Here's how the part is built. I have some questions about the finished solid (model axes, mm). A direction names the side the tool comes from. Round coordinates to 2 decimals unless told otherwise and drop trailing zeros. Order: outer loops, then holes, each group sorted by start corner. A loop starts at its lowest first (then second) coordinate and runs counter-clockwise, first axis right, second up. Notation, with made-up numbers: (53.25, 74.25) -> (111.25, 74.25) arc R10 ccw to (111.25, 91.25) -> close; hole circle Ø3 at (34.25, 29). An arc over 180 degrees is marked (long way). Answer in a Markdown table with one row per item.
```python
from build123d import *

# Parameters (mm, degrees)
F0_W     = 82
F0_H     = 25
F1_DEPTH = 4.5
F2_T     = -1.75
F3_W     = 70.6
F3_H     = 19.5
F4_DEPTH = 50.8
F5_W     = 1
F5_H     = 1.75
F6_DEPTH = 19.49958
F7_W     = 15.24
F7_H     = 5.5
F8_DEPTH = 1.75006


with BuildPart() as f1:
    # F0 (on Front) → F1 (new body)
    with BuildSketch(Plane.XZ):
        Rectangle(F0_W, F0_H)
    extrude(amount=F1_DEPTH)

    # F2
    f2_openings = [f1.faces().sort_by_distance(p)[0] for p in [
        (0, -2.25, 12.5),
    ]]
    offset(amount=F2_T, openings=f2_openings)

    # F3 (on face) → F4 (cut)
    with BuildSketch(Plane.XZ.offset(4.5)):
        with Locations((0, 2.75)):
            Rectangle(F3_W, F3_H)
    extrude(amount=-F4_DEPTH, mode=Mode.SUBTRACT)

    # F5 (on face) → F6 (cut)
    with BuildSketch(Plane.XY.offset(12.5)):
        with Locations((-35.8, -0.875)):
            Rectangle(F5_W, F5_H)
    extrude(amount=-F6_DEPTH, mode=Mode.SUBTRACT)

    # F7 (on face) → F8 (cut)
    with BuildSketch(Plane.XZ.offset(4.5)):
        with Locations((26.41, -9.75)):
            Rectangle(F7_W, F7_H)
    extrude(amount=-F8_DEPTH, mode=Mode.SUBTRACT)


solid = f1.part
```
1. For faces 4 (the face through (34.03, -4, -10)), 5 (the face through (-19, -2.75, -8)), 6 (the face through (-9, -4, -7)), 7 (the face through (-36.3, -1, 3)), which set-ups out of +Z, -Z, +X, -X, +Y, -Y let a thin tool reach every point of the face, with its end or its side?
Numbers:
| item | result |
|---|---|
| face 4 | +Z, -Z, -Y |
| face 5 | +Z |
| face 6 | +Z, +Y, -Y |
| face 7 | +Z, +Y |
2. Suppose I cut it at A-A on z = -2.25. Write out the boundary of the cut face in (x, y).
Numbers:
| item | result |
|---|---|
| outline | (-41, -4.5) -> (-35.3, -4.5) -> (-35.3, -2.75) -> (-39.25, -2.75) -> (-39.25, -1.75) -> (-36.3, -1.75) -> (-36.3, 0) -> (-41, 0) -> close; (35.3, -4.5) -> (41, -4.5) -> (41, 0) -> (35.3, 0) -> (35.3, -1.75) -> (39.25, -1.75) -> (39.25, -2.75) -> (35.3, -2.75) -> close |
3. Suppose I cut it at B-B on x = 1.5. Write out the boundary of the cut face in (y, z), then the cut area to 3 significant figures.
Numbers:
| item | result |
|---|---|
| outline | (-4.5, -12.5) -> (0, -12.5) -> (0, -7) -> (-1.75, -7) -> (-1.75, -10.75) -> (-2.75, -10.75) -> (-2.75, -7) -> (-4.5, -7) -> close |
| area | 21.0 mm2 |
4. We'd pull the mould along X, two halves only. Please class faces 1 (the face through (35.3, -4, 3)), 2 (the face through (41, -2, 0)), 3 (the face through (38, -1, 12.5)): released by +X, released by -X, zero draft, split by the parting line, or undercut.
Numbers:
| item | result |
|---|---|
| face 1 | undercut |
| face 2 | released by +X |
| face 3 | zero draft |
5. Suppose I cut it at C-C on z = -8.75. Write out the boundary of the cut face in (x, y).
Numbers:
| item | result |
|---|---|
| outline | (-41, -4.5) -> (18.79, -4.5) -> (18.79, -2.75) -> (-39.25, -2.75) -> (-39.25, -1.75) -> (39.25, -1.75) -> (39.25, -2.75) -> (34.03, -2.75) -> (34.03, -4.5) -> (41, -4.5) -> (41, 0) -> (-41, 0) -> close |
6. Please list where these lines run through material, in increasing order: line 1 along X through (y, z) = (-3.25, -6.75); line 2 along X through (y, z) = (-0.55, -4.5); line 3 along Z through (x, y) = (26.5, -1.4).
Numbers:
| item | result |
|---|---|
| line 1 | x = -41 to -35.3, 35.3 to 41 |
| line 2 | x = -41 to -36.3, 35.3 to 41 |
| line 3 | z = -12.5 to -7 |
7. For pin 1 Ø6 at (x, z) = (-19.5, -2.5) entering from +Y; pin 2 Ø0.5 at (x, y) = (-35.5, -1) entering from +Z; pin 3 Ø1.4 at (x, z) = (29, -11.5) entering from -Y, each with a flat end and sliding along its axis, tell me the tip position at first contact or that it passes through.
Numbers:
| item | result |
|---|---|
| pin 1 | passes through |
| pin 2 | stops at z = -7 |
| pin 3 | stops at y = -2.75 |
8. Suppose I cut it at D-D on x = 22. Write out the boundary of the cut face in (y, z).
Numbers:
| item | result |
|---|---|
| outline | (-2.75, -12.5) -> (0, -12.5) -> (0, -7) -> (-1.75, -7) -> (-1.75, -10.75) -> (-2.75, -10.75) -> close |
